Autodesk Inventor part; units mm, degrees
ref_plane "YZ Plane" through (0, 0, 0) normal (1, 0, 0) x (0, 1, 0)
ref_plane "XZ Plane" through (0, 0, 0) normal (0, 1, 0) x (-1, 0, 0)
ref_plane "XY Plane" through (0, 0, 0) normal (0, 0, 1) x (1, 0, 0)
sketch "Sketch1" plane through (0, 0, 0) normal (0, 1, 0) x (-1, 0, 0)
  line L0 (-21, 21) -> (21, 21)
  line L1 (21, 21) -> (21, -21)
  line L2 (21, -21) -> (-21, -21)
  line L3 (-21, -21) -> (-21, 21)
  line L4 (-21, 21) -> (21, -21) construction
  line L5 (21, 21) -> (-21, -21) construction
  point P0 (0, 0)
  dimension "d0" = 42
  dimension "d1" = 42
extrude "Extrusion1" add sketch "Sketch1" along normal blind 48
sketch "Sketch2" plane through (0, 48, 0) normal (0, 1, 0) x (1, 0, 0)
  line L0 (21, 21) -> (-21, 21)
  line L1 (-21, 21) -> (-21, -21)
  line L2 (-21, -21) -> (21, -21)
  line L3 (21, -21) -> (21, 21)
  circle A0 centre (0, 0) radius 11
  dimension "d4" = 22
extrude "Extrusion2" add sketch "Sketch2" along normal blind 2 contours A0
sketch "Sketch3" plane through (0, 50, 0) normal (0, 1, 0) x (1, 0, 0)
  circle A0 centre (0, 0) radius 2.5
  dimension "d7" = 5
extrude "Extrusion3" add sketch "Sketch3" along normal blind 22
sketch "Sketch4" plane through (0, 48, 0) normal (0, 1, 0) x (1, 0, 0)
  circle A0 centre (0, 0) radius 2.5
  circle A1 centre (0, 0) radius 2.5
  circle A2 centre (0, 0) radius 11
  line L0 (15.5, -15.5) -> (-15.5, -15.5)
  line L1 (-15.5, -15.5) -> (-15.5, 15.5)
  line L2 (-15.5, 15.5) -> (15.5, 15.5)
  line L3 (15.5, 15.5) -> (15.5, -15.5)
  line L4 (15.5, -15.5) -> (-15.5, 15.5) construction
  line L5 (-15.5, -15.5) -> (15.5, 15.5) construction
  circle A3 centre (-15.5, 15.5) radius 1.5
  circle A4 centre (-15.5, -15.5) radius 1.5
  circle A5 centre (15.5, -15.5) radius 1.5
  circle A6 centre (15.5, 15.5) radius 1.5
  dimension "d10" = 31
  dimension "d11" = 31
  dimension "d12" = 3
  dimension "d15" = 360
extrude "Extrusion4" cut sketch "Sketch4" against normal blind 5 contours A4 L1 L0 | L0 L1 A4 | A5 L3 L0 | L0 L3 A5 | A3 L2 L1 | L1 L2 A3 | A6 L2 L3 | L3 L2 A6
properties part number "Stepper"
Verification items for the finished model (mm, model axes). A direction names the side the tool comes from. Coordinates: 2 decimals unless noted, no trailing zeros. Write each loop counter-clockwise with the first axis right and the second up, starting at its lowest first coordinate (ties: lowest second). Pieces come first, ordered by that corner, then holes. Notation, with made-up numbers: M 38.5,-17.75 L 71.5,-17.75 A29 cw 71.5,7.25 Z; hole C 71.5,-6 d7. An arc over 180 degrees is marked long. One line per question, with ' | ' between items.
1) Sectioned sample at B-B on z = -15.5. Record the cut outline in (x, y), then the cut area to 3 significant figures.
Solutions:
outline: M -21,0 L 21,0 L 21,48 L 17,48 L 17,43 L 14,43 L 14,48 L -14,48 L -14,43 L -17,43 L -17,48 L -21,48 Z | area: 1,990 mm^2
2) Sectioned sample at C-C on y = 60. Record the cut outline in (x, z), then the cut area to 3 significant figures.
Solutions:
outline: C 0,0 d5 | area: 19.6 mm^2
3) Sectioned sample at A-A on x = 0. Record the cut outline in (y, z).
Solutions:
outline: M 0,-21 L 48,-21 L 48,-11 L 50,-11 L 50,-2.5 L 72,-2.5 L 72,2.5 L 50,2.5 L 50,11 L 48,11 L 48,21 L 0,21 Z
4) Sectioned sample at D-D on z = -7.5. Record the cut outline in (x, y), then the cut area to 3 significant figures.
Solutions:
outline: M -21,0 L 21,0 L 21,48 L 8.05,48 L 8.05,50 L -8.05,50 L -8.05,48 L -21,48 Z | area: 2,050 mm^2
5) Access from +Z, -Z, +X, -X, +Y, -Y to the whole of each face (thin tool, end or side, straight path). Record for faces 1 (the face through (-16, 43, -16)), 2 (the face through (-21, 24, 0)).
Solutions:
face 1: +Y | face 2: +Z, -Z, -X, +Y, -Y
6) Depth check by flat-ended pin: pin 1 Ø8 at (x, z) = (13.5, 13) entering from +Y; pin 2 Ø5 at (x, y) = (-3.5, 62) entering from +Z; pin 3 Ø6.5 at (x, z) = (-3, 5.5) entering from +Y. Enter the tip coordinate at first touch or a pass-through.
Solutions:
pin 1: y = 48 | pin 2: z = 2.29 | pin 3: y = 50
7) Release check for a two-part mould opening along X. For faces 3 (the face through (0, 0, 0)), 4 (the face through (21, 24, 0)), 5 (the face through (14, 45.54, 15.43)) record: +X half, -X half, draft (parallel to the pull), parting line (faces both ways), or undercut.
Solutions:
face 3: draft | face 4: +X half | face 5: undercut
8) Material ranges on L1, parallel to Z at x = -15.5, y = 46.8; L2, parallel to Z at x = -15, y = 46, recorded low to high.
Solutions:
L1: -21 to -17, -14 to 14, 17 to 21 | L2: -21 to -16.91, -14.09 to 14.09, 16.91 to 21
